```python
from build123d import *

# Parameters (mm, degrees)
BOSS_EXTRUDE1_DEPTH = 20
FILLET1_R           = 4
SKETCH2_R           = 2.75
CUT_EXTRUDE1_DEPTH  = 1.5
LPATTERN1_COUNT     = 3
LPATTERN1_PITCH     = 30


with BuildPart() as part:
    # Sketch1 → Boss-Extrude1 (new body)
    with BuildSketch(Plane(origin=(0, 0, 0), x_dir=(1, 0, 0), z_dir=(0, 1, 0))):
        with BuildLine():
            Line((37.5, -5), (-37.5, -5))
            ThreePointArc((-37.5, -5), (-42.5, 0), (-37.5, 5))
            Line((-37.5, 5), (37.5, 5))
            ThreePointArc((37.5, 5), (42.5, 0), (37.5, -5))
        make_face()
    extrude(amount=BOSS_EXTRUDE1_DEPTH)

    # Fillet1
    fillet1_edges = [part.edges().sort_by_distance(p)[0] for p in [
        (-42.5, 20, 0),
        (0, 20, 5),
        (42.5, 20, 0),
        (0, 20, -5),
    ]]
    fillet(fillet1_edges, radius=FILLET1_R)

    # Sketch2 → Cut-Extrude1 (cut)
    with BuildSketch(Plane.XZ):
        with Locations(Location((-37.5, 0, 0), (0, 0, 270))):
            Circle(SKETCH2_R)
    cut_extrude1 = extrude(amount=-CUT_EXTRUDE1_DEPTH, mode=Mode.SUBTRACT)

    # LPattern1: Cut-Extrude1 ×3
    with Locations(*[(i * LPATTERN1_PITCH, 0, 0) for i in range(1, LPATTERN1_COUNT)]):
        add(cut_extrude1, mode=Mode.SUBTRACT)


solid = part.part
```
Part model, mm, in its own coordinate system. A direction names the side the tool comes from. Round coordinates to 2 decimals unless told otherwise and drop trailing zeros. Write each loop counter-clockwise with the first axis right and the second up, starting at its lowest first coordinate (ties: lowest second). Pieces come first, ordered by that corner, then holes. Notation, with made-up numbers: M 59,73.25 L 90,73.25 A23 cw 90,97.25 Z; hole C 81.25,38.25 d4. An arc over 180 degrees is marked long. Answer as CSV lines item,"result". Start each with the question number.
1) Drill centre lines: L1, parallel to X at y = 0.75, z = 0; L2, parallel to Y at x = -10, z = 0.5; L3, parallel to X at y = 4, z = -1. Where is each one in solid material? Low to high.
2) Band-saw the part on A-A (x = -7.5). List the corners of the cut face in (y, z), then the cut area to 3 significant figures.
3) Which spindle directions (+Z, -Z, +X, -X, +Y, -Y) get a long thin tool onto all of the face, cutting with end or side? Do faces 4 (the face through (1, 8, 5)), 5 (the face through (-34.773, 0.74, 0.358)). Say none if no direction does.
4) Band-saw the part on B-B (y = 5.25). List the corners of the cut face in (x, z), then the cut area to 3 significant figures.
5) Mould opens along Z. For faces 1 (the face through (1, 0, 0)), 2 (the face through (-10.185, 0.74, 0.596)), 3 (the face through (0.525, 18.797, -3.859)) say: +Z half, -Z half, draft (parallel to the pull), parting line (faces both ways), or undercut.
6) Band-saw the part on D-D (x = 24). List the corners of the cut face in (y, z), then the cut area to 3 significant figures.
7) Drop flat-ended pins along their axis: pin 1 (1.5 mm diameter, centred on x = 11.5, y = 17.5, fed in from -Z); pin 2 (5 mm diameter, centred on x = -7.5, z = 0, fed in from -Y). Give the stop position or say it passes through.
8) Band-saw the part on C-C (x = -17). List the corners of the cut face in (y, z), then the cut area to 3 significant figures.
Worked out:
1,L1,"-42.5 to -40.25, -34.75 to -10.25, -4.75 to 19.75, 25.25 to 42.5"
1,L2,"1.5 to 20"
1,L3,"-42.4 to 42.4"
2,outline,"M 0,-5 L 16,-5 A4 ccw 20,-1 L 20,1 A4 ccw 16,5 L 0,5 L 0,2.75 L 1.5,2.75 L 1.5,-2.75 L 0,-2.75 Z"
2,area,"185 mm²"
3,face 4,"+Z, +X, -X, +Y, -Y"
3,face 5,"-Y"
4,outline,"M -37.5,-5 L 37.5,-5 A5 ccw 37.5,5 L -37.5,5 A5 ccw Z"
4,area,"829 mm²"
5,face 1,"draft"
5,face 2,"undercut"
5,face 3,"-Z half"
6,outline,"M 0,-5 L 16,-5 A4 ccw 20,-1 L 20,1 A4 ccw 16,5 L 0,5 L 0,2.3 L 1.5,2.3 L 1.5,-2.3 L 0,-2.3 Z"
6,area,"186 mm²"
7,pin 1,"z = -4.93"
7,pin 2,"y = 1.5"
8,outline,"M 0,-5 L 16,-5 A4 ccw 20,-1 L 20,1 A4 ccw 16,5 L 0,5 Z"
8,area,"193 mm²"
